from build123d import *

# Parameters (mm, degrees)
F0_R     = 1.5
F1_DEPTH = 50
F2_R     = 5
F3_DEPTH = 25
F4_R     = 1.5


with BuildPart() as f1:
    # F0 (on Front) → F1 (new body)
    with BuildSketch(Plane.XZ):
        Circle(F0_R)
    extrude(amount=-F1_DEPTH)

    # F2 (on Front) → F3 (join)
    with BuildSketch(Plane.XZ):
        Circle(F2_R)
    extrude(amount=F3_DEPTH)

    # F4
    f4_edges = [f1.edges().sort_by_distance(p)[0] for p in [
        (-1.5, 50, 0),
    ]]
    fillet(f4_edges, radius=F4_R)


solid = f1.part
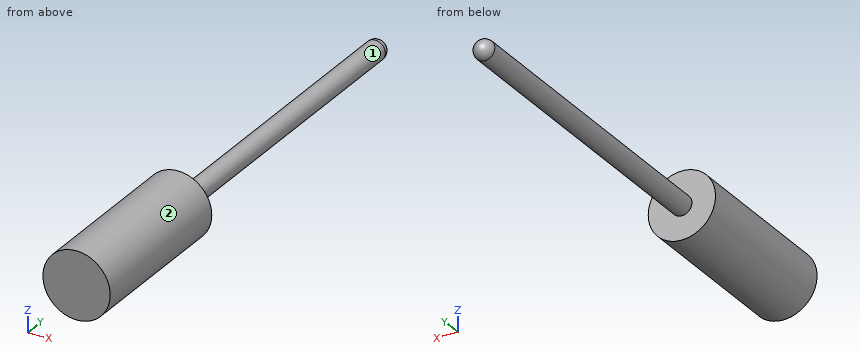
Verification items for the finished model (mm, model axes). Face numbers are marked on the shaded views. A direction names the side the tool comes from. Give positions to 0.01 mm unless a question says otherwise; leave off trailing zeros. Write each loop counter-clockwise with the first axis right and the second up, starting at its lowest first coordinate (ties: lowest second). Pieces come first, ordered by that corner, then holes. Notation, with made-up numbers: M 35,30 L 53,30 A12 cw 53,53 Z; hole C 59.5,-9.75 d11. An arc over 180 degrees is marked long. Put each result on its own line as item: value. Start each with the question number.
1. Section check B-B (x = 0). Record the cut outline in (y, z), and give its area (3 significant figures).
2. Section check D-D (x = -4). Record the cut outline in (y, z), and give its area (3 significant figures).
3. Section check C-C (y = 38). Record the cut outline in (x, z).
4. Section check A-A (z = 0). Record the cut outline in (x, y), and give its area (3 significant figures).
5. Go/stop test with flat-tipped pins: pin 1 Ø1.5 at (x, y) = (-1, 25.5) entering from +Z; pin 2 Ø5 at (x, z) = (-2.5, 1) entering from +Y; pin 3 Ø5 at (x, y) = (-3.5, 8) entering from +Z. Record where each tip stops, or that it passes through.
6. Scan lines: line 1 along Y through (x, z) = (2.5, 3.75); line 2 along Z through (x, y) = (0, 7.5); line 3 along Z through (x, y) = (-4.5, -11). Record each from-to range of solid material in increasing order. Write a range as [from, to].
7. Set-up check for the marked faces 1 and 2: record each of +Z, -Z, +X, -X, +Y, -Y from which the full face is reachable in a straight line by a thin tool's end or side.
Answer list:
1. outline: M -25,-5 L 0,-5 L 0,-1.5 L 48.5,-1.5 A1.5 ccw 48.5,1.5 L 0,1.5 L 0,5 L -25,5 Z
1. area: 399 mm2
2. outline: M -25,-3 L 0,-3 L 0,3 L -25,3 Z
2. area: 150 mm2
3. outline: C 0,0 d3
4. outline: M -5,-25 L 5,-25 L 5,0 L 1.5,0 L 1.5,48.5 A1.5 ccw -1.5,48.5 L -1.5,0 L -5,0 Z
4. area: 399 mm2
5. pin 1: z = 1.48
5. pin 2: y = 49.99
5. pin 3: z = 1.12
6. line 1: [-25, 0]
6. line 2: [-1.5, 1.5]
6. line 3: [-2.18, 2.18]
7. face 1: +Y
7. face 2: +Y, -Y
